The model under review builds one solid part; all positions refer to its coordinate system, in mm. Face numbers are marked on the shaded views. A direction names the side the tool comes from. Coordinates: 2 decimals unless noted, no trailing zeros. Write each loop counter-clockwise with the first axis right and the second up, starting at its lowest first coordinate (ties: lowest second). Pieces come first, ordered by that corner, then holes.
1) Add section B-B, the plane x = 18. State the section outline as (y, z) points, then the cut area to 3 significant figures.
2) Mouldability with a two-part tool opening along X and no side actions: class the marked faces 1 and 2 as released by +X, released by -X, zero draft, split by the parting line, or undercut.
3) For P1, Ø6.5, axis at x = -18.5, z = -9, coming from the +Y side; P2, Ø2, axis at y = 0, z = 69.75, coming from the -X side; P3, Ø2.5, axis at y = 2.5, z = 10, coming from the +X side, all flat-tipped, find the tip position at first contact; note any pin that passes through.
4) Add section C-C, the plane x = -11. State the section outline as (y, z) points.
5) Add section A-A, the plane z = 38.5. State the section outline as (x, y) points, then the cut area to 3 significant figures.
6) Machinability: for the marked faces 3 and 4, which of the approach directions +Z, -Z, +X, -X, +Y, -Y give a long, thin tool a straight path to every point of the face, cutting with its end or side? Answer none if there is none.
7) Add section D-D, the plane x = 0. State the section outline as (y, z) points.
8) For line 1 (Z direction, x = 5, y = -1.75); line 2 (Y direction, x = 30, z = -15.5); line 3 (Z direction, x = 0, y = -1.75), list the stretches that pass through material, from the lowest coordinate up.
from build123d import *

# Parameters (mm, degrees)
SKETCH1_W                                            = 70
SKETCH1_H                                            = 40.5
BOSS_EXTRUDE1_DEPTH                                  = 5
CBORE_FOR_M4_HEXAGON_SOCKET_HEAD_CAP_SCR_D           = 4.5
CBORE_FOR_M4_HEXAGON_SOCKET_HEAD_CAP_SCR_CBORE_D     = 8
CBORE_FOR_M4_HEXAGON_SOCKET_HEAD_CAP_SCR_CBORE_DEPTH = 4.6
CUT_EXTRUDE1_DEPTH                                   = 41.794883258
CUT_EXTRUDE2_DEPTH                                   = 41.794883258
M4_TAPPED_HOLE1_D                                    = 3.3
SKETCH10_W                                           = 10
SKETCH10_H                                           = 30.5
CUT_EXTRUDE3_DEPTH                                   = 42.654081433
SKETCH13_W                                           = 50
SKETCH13_H                                           = 54.5
BOSS_EXTRUDE3_DEPTH                                  = 10
SKETCH14_W                                           = 20
SKETCH14_H                                           = 20
SKETCH14_W_2                                         = 30
SKETCH14_H_2                                         = 45
CUT_EXTRUDE4_DEPTH                                   = 84.141821606
M4_TAPPED_HOLE3_D                                    = 3.3
M4_TAPPED_HOLE3_DEPTH                                = 11.5
M4_TAPPED_HOLE3_TIP                                  = 0.991420021
FILLET1_R                                            = 3
CHAMFER1_SIZE                                        = 2
CHAMFER2_SIZE                                        = 2
CHAMFER3_SIZE                                        = 2


with BuildPart() as part:
    # Sketch1 → Boss-Extrude1 (new, symmetric)
    with BuildSketch(Plane(origin=(0, 0, 0), x_dir=(1, 0, 0), z_dir=(0, 1, 0))):
        Rectangle(SKETCH1_W, SKETCH1_H)
    extrude(amount=BOSS_EXTRUDE1_DEPTH, both=True)

    # CBORE for M4 Hexagon socket head cap screws1 (through all)
    with Locations(Plane(origin=(0, 5, 0), x_dir=(1, 0, 0), z_dir=(0, 1, 0))):
        with Locations((-18, 10.75), (18, 10.75), (18, -10.75), (-18, -10.75)):
            CounterBoreHole(CBORE_FOR_M4_HEXAGON_SOCKET_HEAD_CAP_SCR_D / 2, CBORE_FOR_M4_HEXAGON_SOCKET_HEAD_CAP_SCR_CBORE_D / 2, CBORE_FOR_M4_HEXAGON_SOCKET_HEAD_CAP_SCR_CBORE_DEPTH)

    # Sketch4 → Cut-Extrude1 (cut, through all)
    with BuildSketch(Plane(origin=(0, 0.4, 0), x_dir=(1, 0, 0), z_dir=(0, 1, 0))):
        with BuildLine():
            Line((-22, 8.25), (-22, 13.25))
            ThreePointArc((-22, 13.25), (-18, 17.25), (-14, 13.25))
            Line((-14, 13.25), (-14, 8.25))
            ThreePointArc((-14, 8.25), (-18, 4.25), (-22, 8.25))
        make_face()
        with BuildLine():
            Line((22, 13.25), (22, 8.25))
            ThreePointArc((22, 8.25), (18, 4.25), (14, 8.25))
            Line((14, 8.25), (14, 13.25))
            ThreePointArc((14, 13.25), (18, 17.25), (22, 13.25))
        make_face()
        with BuildLine():
            Line((-14, -8.25), (-14, -13.25))
            ThreePointArc((-14, -13.25), (-18, -17.25), (-22, -13.25))
            Line((-22, -13.25), (-22, -8.25))
            ThreePointArc((-22, -8.25), (-18, -4.25), (-14, -8.25))
        make_face()
        with BuildLine():
            Line((22, -8.25), (22, -13.25))
            ThreePointArc((22, -13.25), (18, -17.25), (14, -13.25))
            Line((14, -13.25), (14, -8.25))
            ThreePointArc((14, -8.25), (18, -4.25), (22, -8.25))
        make_face()
    extrude(amount=CUT_EXTRUDE1_DEPTH, mode=Mode.SUBTRACT)

    # Sketch5 → Cut-Extrude2 (cut, through all)
    with BuildSketch(Plane(origin=(0, 0.4, 0), x_dir=(1, 0, 0), z_dir=(0, 1, 0))):
        with BuildLine():
            Line((-15.75, 13.25), (-15.75, 8.25))
            ThreePointArc((-15.75, 8.25), (-18, 6), (-20.25, 8.25))
            Line((-20.25, 8.25), (-20.25, 13.25))
            ThreePointArc((-20.25, 13.25), (-18, 15.5), (-15.75, 13.25))
        make_face()
        with BuildLine():
            Line((20.25, 13.25), (20.25, 8.25))
            ThreePointArc((20.25, 8.25), (18, 6), (15.75, 8.25))
            Line((15.75, 8.25), (15.75, 13.25))
            ThreePointArc((15.75, 13.25), (18, 15.5), (20.25, 13.25))
        make_face()
        with BuildLine():
            Line((-15.75, -8.25), (-15.75, -13.25))
            ThreePointArc((-15.75, -13.25), (-18, -15.5), (-20.25, -13.25))
            Line((-20.25, -13.25), (-20.25, -8.25))
            ThreePointArc((-20.25, -8.25), (-18, -6), (-15.75, -8.25))
        make_face()
        with BuildLine():
            Line((20.25, -8.25), (20.25, -13.25))
            ThreePointArc((20.25, -13.25), (18, -15.5), (15.75, -13.25))
            Line((15.75, -13.25), (15.75, -8.25))
            ThreePointArc((15.75, -8.25), (18, -6), (20.25, -8.25))
        make_face()
    extrude(amount=-CUT_EXTRUDE2_DEPTH, mode=Mode.SUBTRACT)

    # M4 Tapped Hole1 (through all)
    with Locations(Plane(origin=(0, 0, -20.25), x_dir=(-1, 0, 0), z_dir=(0, 0, -1))):
        with Locations((-30, 0), (30, 0)):
            Hole(M4_TAPPED_HOLE1_D / 2)

    # Sketch10 → Cut-Extrude3 (cut, through all)
    with BuildSketch(Plane(origin=(0, 5, 0), x_dir=(1, 0, 0), z_dir=(0, 1, 0))):
        with Locations((-30, -5)):
            Rectangle(SKETCH10_W, SKETCH10_H)
        with Locations((30, -5)):
            Rectangle(SKETCH10_W, SKETCH10_H)
    extrude(amount=-CUT_EXTRUDE3_DEPTH, mode=Mode.SUBTRACT)

    # Sketch13 → Boss-Extrude3 (add)
    with BuildSketch(Plane(origin=(0, 5, 0), x_dir=(1, 0, 0), z_dir=(0, 1, 0))):
        with Locations((0, -47.5)):
            Rectangle(SKETCH13_W, SKETCH13_H)
    extrude(amount=-BOSS_EXTRUDE3_DEPTH)

    # Sketch14 → Cut-Extrude4 (cut, through all)
    with BuildSketch(Plane(origin=(0, 5, 0), x_dir=(1, 0, 0), z_dir=(0, 1, 0))):
        with Locations((0, 0.25)):
            Rectangle(SKETCH14_W, SKETCH14_H)
        with Locations((0, -42.25)):
            Rectangle(SKETCH14_W_2, SKETCH14_H_2)
    extrude(amount=-CUT_EXTRUDE4_DEPTH, mode=Mode.SUBTRACT)

    # Sketch17 → M4 Tapped Hole2 (revolve, cut)
    with BuildSketch(Plane(origin=(-25, 0, 69.75), x_dir=(0, 0, 1), z_dir=(0, 1, 0))):
        Polygon((0, 0), (0, 12.491420021), (1.65, 11.5), (1.65, 0), align=None)
    m4_tapped_hole2 = revolve(axis=Axis((-31.35, 0, 69.75), (1, 0, 0)), mode=Mode.SUBTRACT)

    # Mirror1: M4 Tapped Hole2 across plane
    add(m4_tapped_hole2.mirror(Plane(origin=(0, 0, 0), x_dir=(0, 0, 1), z_dir=(1, 0, 0))), mode=Mode.SUBTRACT)

    # M4 Tapped Hole3
    with Locations(Plane(origin=(0, 5, 0), x_dir=(1, 0, 0), z_dir=(0, 1, 0))):
        with Locations((0, -69.75)):
            Hole(M4_TAPPED_HOLE3_D / 2, depth=M4_TAPPED_HOLE3_DEPTH)
            with Locations((0, 0, -(M4_TAPPED_HOLE3_DEPTH + M4_TAPPED_HOLE3_TIP / 2))):  # 118° drill point
                Cone(0, M4_TAPPED_HOLE3_D / 2, M4_TAPPED_HOLE3_TIP, mode=Mode.SUBTRACT)

    # Fillet1
    fillet1_edges = [part.edges().sort_by_distance(p)[0] for p in [
        (-25, 0, -10.25),
        (25, 0, -10.25),
        (-10, 0, 9.75),
        (-10, 0, -10.25),
        (10, 0, -10.25),
        (10, 0, 9.75),
        (-15, 0, 19.75),
        (15, 0, 19.75),
        (15, 0, 64.75),
        (-15, 0, 64.75),
    ]]
    fillet(fillet1_edges, radius=FILLET1_R)

    # Chamfer1
    chamfer1_edges = [part.edges().sort_by_distance(p)[0] for p in [
        (-35, 0, -10.25),
        (35, 0, -10.25),
    ]]
    chamfer(chamfer1_edges, length=CHAMFER1_SIZE)

    # Chamfer2
    chamfer2_edges = [part.edges().sort_by_distance(p)[0] for p in [
        (35, 5, -16.25),
        (-35, 5, -16.25),
    ]]
    chamfer(chamfer2_edges, length=CHAMFER2_SIZE)

    # Chamfer3
    chamfer3_edges = [part.edges().sort_by_distance(p)[0] for p in [
        (-30.5, -5, -10.25),
        (-25.878679656, -5, -9.371320344),
        (-25, -5, 33.75),
        (30.5, -5, -10.25),
        (25.878679656, -5, -9.371320344),
        (25, -5, 33.75),
    ]]
    chamfer(chamfer3_edges, length=CHAMFER3_SIZE)


solid = part.part
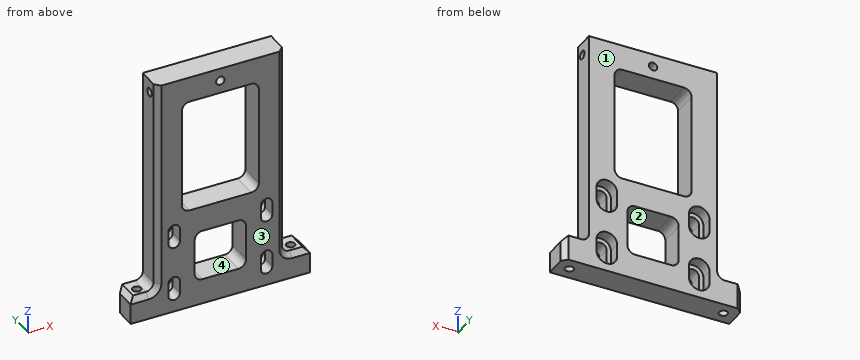
Geometry results:
1. outline: (-5, -20.25) - (5, -20.25) - (5, -17.25) - (0.4, -17.25) - (0.4, -15.5) - (-5, -15.5) - close; (-5, -6) - (0.4, -6) - (0.4, -4.25) - (5, -4.25) - (5, 4.25) - (0.4, 4.25) - (0.4, 6) - (-5, 6) - close; (-5, 15.5) - (0.4, 15.5) - (0.4, 17.25) - (5, 17.25) - (5, 74.75) - (-5, 74.75) - close; hole circle Ø3.3 at (0, 69.75)
1. area: 719 mm2
2. face 1: zero draft
2. face 2: undercut
3. P1: stops at y = 0.4
3. P2: stops at x = -13.11
3. P3: stops at x = 25
4. outline: (-5, -20.25) - (5, -20.25) - (5, 19.75) - (-5, 19.75) - close; (-5, 64.75) - (5, 64.75) - (5, 74.75) - (-5, 74.75) - close
5. outline: (-25, -3) - (-23, -5) - (-15, -5) - (-15, 5) - (-25, 5) - close; (15, -5) - (23, -5) - (25, -3) - (25, 5) - (15, 5) - close
5. area: 196 mm2
6. face 3: +Z, -Z, +X, -X, -Y
6. face 4: +Y, -Y
7. outline: (-5, -20.25) - (5, -20.25) - (5, -10.25) - (-5, -10.25) - close; (-5, 9.75) - (5, 9.75) - (5, 19.75) - (-5, 19.75) - close; (-5, 64.75) - (5, 64.75) - (5, 68.1) - (-5, 68.1) - close; (-5, 71.4) - (5, 71.4) - (5, 74.75) - (-5, 74.75) - close
8. line 1: z = -20.25 to -10.25, 9.75 to 19.75, 64.75 to 74.75
8. line 2: y = -5 to -1.65, 1.65 to 5
8. line 3: z = -20.25 to -10.25, 9.75 to 19.75, 64.75 to 68.1, 71.4 to 74.75
